Read the model definition and answer for the solid it produces. Units are mm, in the model's axes. Give positions to 0.01 mm unless a question says otherwise; leave off trailing zeros. Order: outer loops, then holes, each group sorted by start corner. A loop starts at its lowest first (then second) coordinate and runs counter-clockwise, first axis right, second up.
Autodesk Inventor part; units mm, degrees
ref_plane "YZ Plane" through (0, 0, 0) normal (1, 0, 0) x (0, 1, 0)
ref_plane "XZ Plane" through (0, 0, 0) normal (0, 1, 0) x (-1, 0, 0)
ref_plane "XY Plane" through (0, 0, 0) normal (0, 0, 1) x (1, 0, 0)
sketch "Sketch1" plane through (0, 0, 0) normal (0, 0, 1) x (1, 0, 0)
  arc A0 (6.3455, 7.6592) -> (2.9969, 4.161) centre (5.1207, 5.4798) ccw
  arc A1 (28.9309, -45.2636) -> (10.279, 5.1864) centre (-16.779, -33.4901) ccw
  arc A2 (8.9309, -45.2636) -> (6.4804, -0.2246) centre (-28.4708, -24.7125) ccw
  line L0 (8.9309, -45.2636) -> (28.9309, -45.2636)
  arc A3 (2.9969, 4.161) -> (6.4804, -0.2246) centre (4.7985, 2.0157) ccw
  arc A4 (10.279, 5.1864) -> (5.805, 7.8843) centre (7.5999, 5.8022) ccw
  circle A5 centre (20.9309, -38.1135) radius 2
  point P0 (0, 0)
  dimension "d25" = 2.5
  dimension "d32" = 20
  dimension "d50" = 7.1502
  dimension "d51" = 8
extrude "Extrusion4" add sketch "Sketch1" along normal blind 5
fillet "Fillet3" radius 7 2 edges at (8.9309, -45.2636, 2.5) (28.9309, -45.2636, 2.5)
properties part number "mavac_ruka I guesss"
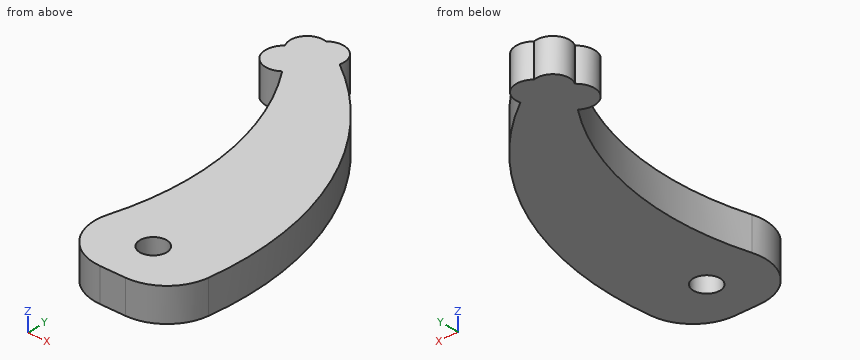
1) The part is cut by section A-A on z = 4. Determine the outline of the cut face in (x, y) (1 decimal), and give its area (3 significant figures).
Final values:
outline: (3, 4.2) arc R2.8 ccw to (6.5, -0.2) arc R42.7 cw to (12.6, -36.4) arc R7 ccw to (19.3, -45.3) - (23.1, -45.3) arc R7 ccw to (30.1, -39.1) arc R47.2 ccw to (10.3, 5.2) arc R2.7 ccw to (5.8, 7.9) arc R2.5 ccw to start; hole circle Ø4 at (20.9, -38.1)
area: 719 mm2
2) Consider L1, parallel to Y at x = 5, z = 0.75; L2, parallel to X at y = -29, z = 1.6; L3, parallel to X at y = -41, z = 1.6. Determine where each line is inside the solid, lowest interval first.
Final values:
L1: y = -0.78 to 7.98
L2: x = 13.99 to 30.21
L3: x = 12.88 to 29.58
3) Given pin 1 (1.5 mm diameter, centred on y = -31, z = 4, fed in from -X); pin 2 (2 mm diameter, centred on y = -0.5, z = 3, fed in from +X), each flat-ended and moving along its own axis, determine where each tip first touches the part or whether it passes through.
Final values:
pin 1: stops at x = 13.62
pin 2: stops at x = 17.93
4) The part is cut by section C-C on x = 9.75. Determine the outline of the cut face in (y, z).
Final values:
outline: (-5.73, 0) - (7.52, 0) - (7.52, 5) - (-5.73, 5) - close
5) The part is cut by section B-B on y = -22.5. Determine the outline of the cut face in (x, z), and give its area (3 significant figures).
Final values:
outline: (14.15, 0) - (29.13, 0) - (29.13, 5) - (14.15, 5) - close
area: 74.9 mm2
